Check sheet for the modelled part. Datum: model origin and axes. Units: mm. Face numbers are marked on the shaded views. A direction names the side the tool comes from. Round coordinates to 2 decimals unless told otherwise and drop trailing zeros. Write each loop counter-clockwise with the first axis right and the second up, starting at its lowest first coordinate (ties: lowest second). Pieces come first, ordered by that corner, then holes.
Item 1: Go/stop test with flat-tipped pins: pin 1 Ø3 at (x, z) = (-8, 3) entering from -Y; pin 2 Ø2 at (x, z) = (-2, 2.5) entering from +Y. Record where each tip stops, or that it passes through.
Item 2: Cross-section at D-D on y = -6.75. Enter the section's corners in (x, z), plus the area to 3 significant figures.
Item 3: Release check for a two-part mould opening along Y. For the marked faces 4, 5 and 6 record: +Y half, -Y half, draft (parallel to the pull), parting line (faces both ways), or undercut.
Item 4: Tool access check on the marked faces 1, 2 and 3. Record the directions out of +Z, -Z, +X, -X, +Y, -Y that give a thin tool (end or side, any length) a straight path to the whole face; none if there is none.
Item 5: Cross-section at A-A on z = 1.05. Enter the section's corners in (x, y), plus the area to 3 significant figures.
Item 6: Material ranges on line 1 (Z direction, x = -2.25, y = -5); line 2 (X direction, y = -10.25, z = 3.3); line 3 (Z direction, x = -3.5, y = -4.5), recorded low to high.
Item 7: Cross-section at C-C on z = 2.15. Enter the section's corners in (x, y), plus the area to 3 significant figures.
Item 8: Cross-section at B-B on z = 0.3. Enter the section's corners in (x, y), plus the area to 3 significant figures.
from build123d import *

# Parameters (mm, degrees)
BOSS_EXTRUDE1_DEPTH = 5.08
FILLET1_R           = 0.762
SKETCH2_R           = 1.905
CUT_EXTRUDE1_DEPTH  = 10.53526285


with BuildPart() as part:
    # Sketch1 → Boss-Extrude1 (new body)
    with BuildSketch(Plane.XY):
        Polygon((0, 0), (-10.367708313, -4.812018738), (-7.286004456, -6.993932896), (-9.487605847, -10.103442715), (-6.378096028, -12.305044107), (-4.176494637, -9.195534288), (-1.020567729, -11.43), align=None)
    extrude(amount=BOSS_EXTRUDE1_DEPTH)

    # Fillet1
    fillet1_edges = [part.edges().sort_by_distance(p)[0] for p in [
        (-1.020567729, -11.43, 2.54),
        (-6.378096028, -12.305044107, 2.54),
        (-9.487605847, -10.103442715, 2.54),
        (-10.367708313, -4.812018738, 2.54),
        (0, 0, 2.54),
    ]]
    fillet(fillet1_edges, radius=FILLET1_R)

    # Sketch2 → Cut-Extrude1 (cut, through all)
    with BuildSketch(Plane(origin=(0, 0, 0), x_dir=(0, 0, -1), z_dir=(0.996037458, -0.088934706, 0))):
        with Locations((-2.54, -4.367822715)):
            Circle(SKETCH2_R)
    extrude(amount=-CUT_EXTRUDE1_DEPTH, mode=Mode.SUBTRACT)


solid = part.part
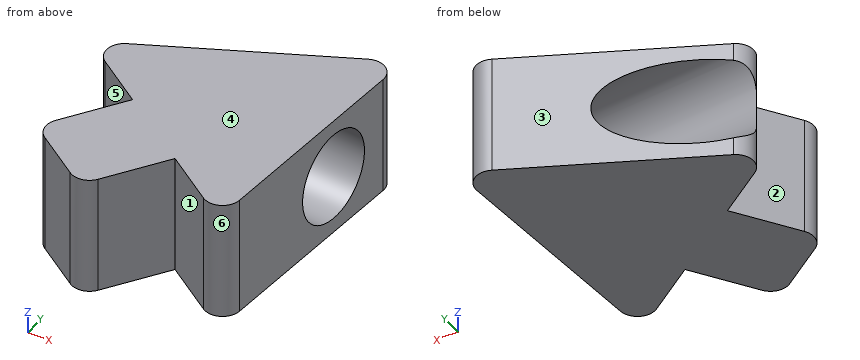
Response values:
1. pin 1: stops at y = -12
1. pin 2: stops at y = -0.49
2. outline: (-7.63, 0) - (-0.6, 0) - (-0.6, 5.08) - (-7.63, 5.08) - close
2. area: 35.7 mm2
3. face 4: draft
3. face 5: undercut
3. face 6: -Y half
4. face 1: +Z, -Z, -Y
4. face 2: +Z, -Z, -X
4. face 3: +Z, -Z, -X, +Y
5. outline: (-9.58, -4.72) arc R0.76 ccw to (-9.29, -5.57) - (-7.29, -6.99) - (-9.05, -9.48) arc R0.76 ccw to (-8.87, -10.54) - (-7, -11.86) arc R0.76 ccw to (-5.94, -11.68) - (-4.18, -9.2) - (-2.1, -10.66) arc R0.76 ccw to (-0.9, -10.11) - (-0.49, -5.53) - close; (-5.77, -2.68) - (-0.28, -3.17) - (-0.12, -1.31) arc R0.76 ccw to (-1.2, -0.56) - close
5. area: 52.0 mm2
6. line 1: z = 0 to 0.82, 4.26 to 5.08
6. line 2: x = -9.11 to -4.92, -2.69 to -0.93
6. line 3: z = 0 to 0.68, 4.4 to 5.08
7. outline: (-9.46, -5.41) arc R0.76 ccw to (-9.29, -5.57) - (-7.29, -6.99) - (-9.05, -9.48) arc R0.76 ccw to (-8.87, -10.54) - (-7, -11.86) arc R0.76 ccw to (-5.94, -11.68) - (-4.18, -9.2) - (-2.1, -10.66) arc R0.76 ccw to (-0.9, -10.11) - (-0.55, -6.21) - close; (-4.54, -2.11) - (-0.22, -2.49) - (-0.12, -1.31) arc R0.76 ccw to (-1.2, -0.56) - close
7. area: 42.5 mm2
8. outline: (-9.29, -5.57) - (-7.29, -6.99) - (-9.05, -9.48) arc R0.76 ccw to (-8.87, -10.54) - (-7, -11.86) arc R0.76 ccw to (-5.94, -11.68) - (-4.18, -9.2) - (-2.1, -10.66) arc R0.76 ccw to (-0.9, -10.11) - (-0.12, -1.31) arc R0.76 ccw to (-1.2, -0.56) - (-9.18, -4.26) arc R0.76 ccw to start
8. area: 69.9 mm2
